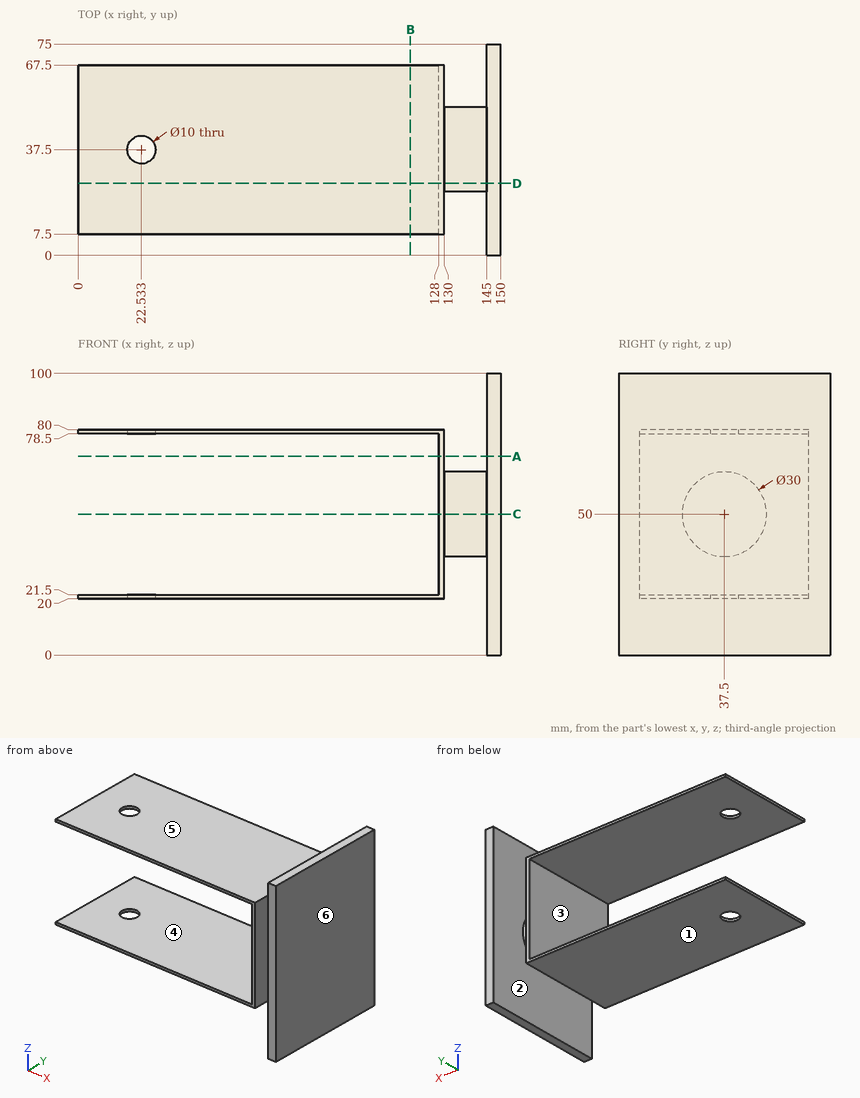
Can you work these out from the drawing? Everything is in mm from the part's minimum corner. A direction names the side the tool comes from. Coordinates: 2 decimals unless noted, no trailing zeros. Loops run counter-clockwise (first coordinate to the right, second up) from the corner with the lowest first, then second, coordinate; pieces in that order, holes last.
1. If we mould it in two halves opening along Z, with no side actions, what happens to the marked faces 1, 2 and 3? For each: pulls with the +Z half, pulls with the -Z half, needs draft (parallel to the pull), parting line crosses it, or undercut.
2. Imagine slicing it at D-D, the plane y = 25.5. Please give me the cut outline in (x, z), and give its area (3 significant figures).
3. Imagine slicing it at C-C, the plane z = 50. Please give me the cut outline in (x, y).
4. For the marked faces 4, 5 and 6, which set-ups out of +Z, -Z, +X, -X, +Y, -Y let a thin tool reach every point of the face, with its end or its side?
5. Imagine slicing it at A-A, the plane z = 70.5. Please give me the cut outline in (x, y), and give its area (3 significant figures).
6. Imagine slicing it at B-B, the plane x = 118. Please give me the cut outline in (y, z).
7. I need wall thicknesses on L1, parallel to X at y = 37.5, z = 79.1; L2, parallel to Z at x = 97.5, y = 35.5; L3, parallel to X at y = 37.5, z = 77.5. Which ranges of each line are inside material? Lowest first, please.
8. For P1, Ø1, axis at x = 36.5, z = 21, coming from the -Y side; P2, Ø12, axis at x = 124.5, z = 53.5, coming from the +Y side; P3, Ø11.5, axis at x = 22.53, y = 37.5, coming from the +Z side; P4, Ø22.5, axis at y = 42, z = 29, coming from the -X side, each with a flat end and sliding along its axis, tell me the tip position at first contact or that it passes through.
Taken from the geometry:
1. face 1: pulls with the -Z half
1. face 2: needs draft
1. face 3: undercut
2. outline: (0, 20) - (130, 20) - (130, 41) - (145, 41) - (145, 0) - (150, 0) - (150, 100) - (145, 100) - (145, 59) - (130, 59) - (130, 80) - (0, 80) - (0, 78.5) - (128, 78.5) - (128, 21.5) - (0, 21.5) - close
2. area: 1,270 mm2
3. outline: (128, 7.5) - (130, 7.5) - (130, 22.5) - (145, 22.5) - (145, 0) - (150, 0) - (150, 75) - (145, 75) - (145, 52.5) - (130, 52.5) - (130, 67.5) - (128, 67.5) - close
4. face 4: -X, +Y, -Y
4. face 5: +Z, -X, +Y, -Y
4. face 6: +Z, -Z, +X, +Y, -Y
5. outline: (128, 7.5) - (130, 7.5) - (130, 67.5) - (128, 67.5) - close; (145, 0) - (150, 0) - (150, 75) - (145, 75) - close
5. area: 495 mm2
6. outline: (7.5, 20) - (67.5, 20) - (67.5, 21.5) - (7.5, 21.5) - close; (7.5, 78.5) - (67.5, 78.5) - (67.5, 80) - (7.5, 80) - close
7. L1: x = 0 to 17.53, 27.53 to 130, 145 to 150
7. L2: z = 20 to 21.5, 78.5 to 80
7. L3: x = 128 to 130, 145 to 150
8. P1: stops at y = 7.5
8. P2: stops at y = 67.5
8. P3: stops at z = 80
8. P4: stops at x = 0
